from build123d import *

# Parameters (mm, degrees)
SKETCH1_W           = 25
SKETCH1_H           = 45
SKETCH1_R           = 1.375
BOSS_EXTRUDE1_DEPTH = 2.54
FILLET1_R           = 2.54


with BuildPart() as part:
    # Sketch1 → Boss-Extrude1 (new body)
    with BuildSketch(Plane.XY):
        with Locations((12.5, -22.5)):
            Rectangle(SKETCH1_W, SKETCH1_H)
        with Locations((2.75, -2.75)):
            Circle(SKETCH1_R, mode=Mode.SUBTRACT)
        with Locations((2.75, -42.25)):
            Circle(SKETCH1_R, mode=Mode.SUBTRACT)
        with Locations((22.25, -42.25)):
            Circle(SKETCH1_R, mode=Mode.SUBTRACT)
        with Locations((22.25, -2.75)):
            Circle(SKETCH1_R, mode=Mode.SUBTRACT)
    extrude(amount=BOSS_EXTRUDE1_DEPTH)

    # Fillet1
    fillet1_edges = [part.edges().sort_by_distance(p)[0] for p in [
        (0, 0, 1.27),
        (25, 0, 1.27),
        (25, -45, 1.27),
        (0, -45, 1.27),
    ]]
    fillet(fillet1_edges, radius=FILLET1_R)


solid = part.part
Source: CAD feature listing. Evaluate the final solid. Frame: model axes, mm. Round coordinates to 2 decimals unless told otherwise and drop trailing zeros. Loops run counter-clockwise (first coordinate to the right, second up) from the corner with the lowest first, then second, coordinate; pieces in that order, holes last. Notation, with made-up numbers: (-30.5, 17) - (15.5, 17) arc R23 ccw to (15.5, 53) - close; hole circle Ø8 at (-35, -18). An arc over 180 degrees is marked (long way). Write item = value, one per line. Start each with the question number.
(1) Pin query (flat end, axial travel): pin 1 (1.6 mm diameter, centred on x = 2.75, y = -2.75, fed in from +Z). Return the tip coordinate at first contact, or that it passes through.
(2) Pull-direction query (X, two-part tool) for faces 1 (the face through (25, -23, 1)), 2 (the face through (0, -23, 1)), 3 (the face through (4.062, -41.837, 1.252)), 4 (the face through (12, -22, 0)); classes: +X half, -X half, draft (parallel to the pull), parting line (faces both ways), or undercut.
(3) Ray query, line 1 along Y through (x, z) = (2.75, 0.8) (3 decimals); line 2 along Y through (x, z) = (21.5, 2.25). Return the intervals inside material, ascending. Write a range as from..to.
(4) Section query A-A, the plane z = 1. Output: boundary loops of the cut face in (x, y) (3 decimals).
Conclusion:
q1.pin_1 = through
q2.face_1 = +X half
q2.face_2 = -X half
q2.face_3 = undercut
q2.face_4 = draft
q3.line_1 = -45..-43.625, -40.875..-4.125, -1.375..0
q3.line_2 = -45..-43.4, -41.1..-3.9, -1.6..0
q4.outline = (0, -42.46) arc R2.54 ccw to (2.54, -45) - (22.46, -45) arc R2.54 ccw to (25, -42.46) - (25, -2.54) arc R2.54 ccw to (22.46, 0) - (2.54, 0) arc R2.54 ccw to (0, -2.54) - close; hole circle Ø2.75 at (2.75, -42.25); hole circle Ø2.75 at (2.75, -2.75); hole circle Ø2.75 at (22.25, -42.25); hole circle Ø2.75 at (22.25, -2.75)
